Verification items for the finished model (mm, model axes). A direction names the side the tool comes from. Round coordinates to 2 decimals unless told otherwise and drop trailing zeros. Order: outer loops, then holes, each group sorted by start corner. A loop starts at its lowest first (then second) coordinate and runs counter-clockwise, first axis right, second up. Notation, with made-up numbers: (12, -28) -> (62, -28) arc R32 cw to (62, -1) -> close; hole circle Ø4 at (-26, -25). An arc over 180 degrees is marked (long way). Return JSON: item names as keys, results as strings. Group by question number.
Item 1: Sectioned sample at A-A on z = 10. Record the cut outline in (x, y), plus the area to 3 significant figures.
Item 2: Access from +Z, -Z, +X, -X, +Y, -Y to the whole of each face (thin tool, end or side, straight path). Record for faces 5 (the flat face through (-47.5, -90, -31)), 6 (the flat face through (-45, -41, -30)), 7 (the flat face through (47.5, -90, -31)), 8 (the flat face through (0, -95, 1)), 9 (the flat face through (40, -3, -20)).
Item 3: Draft check along X on faces 1 (the flat face through (75, -3, 3)), 2 (the flat face through (-1, -175, -35)), 3 (the flat face through (-1, -172, -35)), 4 (the flat face through (42.5, -79, -27)). Enter one of: pulls with the +X half, pulls with the -X half, needs draft (parallel to the pull), parting line crosses it, or undercut.
Item 4: Depth check by flat-ended pin: pin 1 Ø5.5 at (x, y) = (-46, -58) entering from +Z; pin 2 Ø1.5 at (x, z) = (35, 0) entering from +Y; pin 3 Ø20 at (x, y) = (11.5, -87.5) entering from -Z. Enter the tip coordinate at first touch or a pass-through.
Item 5: Sectioned sample at B-B on y = -98. Record the cut outline in (x, z).
Item 6: Scan lines: probe 1 along X at (y, z) = (-3.8, -32); probe 2 along Z at (x, y) = (-69, -2.2); probe 3 along Y at (x, z) = (45, -11). Record each from-to range of solid material in increasing order. Write a range as from..to.
```python
from build123d import *

# Parameters (mm, degrees)
F0_W     = 5
F0_H     = 3
F0_H_2   = 30
F1_DEPTH = 6
F0_H_3   = 10
F2_DEPTH = 175
F3_DEPTH = 3
F4_START = 172
F0_W_2   = 75
F4_DEPTH = 3
F5_START = 77
F5_DEPTH = 18
F6_D     = 2


# Not quite as in the source:
# - a feature names something its author has since deleted; it is built from what else it names


with BuildPart() as f1:
    # F0 (on Front) → F1 (new body)
    with BuildSketch(Plane.XZ):
        Polygon((75, 48), (-75, 48), (-75, -40), (-47.5, -40), (-47.5, -30), (-47.5, 0), (-47.5, 3), (-42.5, 3), (-42.5, 36), (42.5, 36), (75, 36), align=None)
        Polygon((75, -40), (75, 36), (42.5, 36), (42.5, 3), (47.5, 3), (47.5, 0), (47.5, -30), (47.5, -40), align=None)
        with Locations((45, 1.5)):
            Rectangle(F0_W, F0_H)
        with Locations((45, -15)):
            Rectangle(F0_W, F0_H_2)
        with Locations((-45, 1.5)):
            Rectangle(F0_W, F0_H)
        with Locations((-45, -15)):
            Rectangle(F0_W, F0_H_2)
    extrude(amount=F1_DEPTH)

    # F0 (on Front) → F2 (join)
    with BuildSketch(Plane.XZ):
        with Locations((-45, -35)):
            Rectangle(F0_W, F0_H_3)
        with Locations((45, -35)):
            Rectangle(F0_W, F0_H_3)
    extrude(amount=F2_DEPTH)

    # F0 (on Front) → F3 (join)
    with BuildSketch(Plane.XZ):
        with Locations((-40, -15)):
            Rectangle(F0_W, F0_H_2)
        with Locations((-40, -35)):
            Rectangle(F0_W, F0_H_3)
        with Locations((40, -35)):
            Rectangle(F0_W, F0_H_3)
        with Locations((40, -15)):
            Rectangle(F0_W, F0_H_2)
    extrude(amount=F3_DEPTH)

    # F0 (on Front) → F4 (join)
    with BuildSketch(Plane.XZ.offset(F4_START)):
        with Locations((-40, -35)):
            Rectangle(F0_W, F0_H_3)
        with Locations((40, -35)):
            Rectangle(F0_W, F0_H_3)
        with Locations((0, -35)):
            Rectangle(F0_W_2, F0_H_3)
    extrude(amount=F4_DEPTH)

    # F0 (on Front) → F5 (join)
    with BuildSketch(Plane.XZ.offset(F5_START)):
        with Locations((-45, -15)):
            Rectangle(F0_W, F0_H_2)
        with Locations((45, -15)):
            Rectangle(F0_W, F0_H_2)
        Polygon((42.5, 0), (42.5, 3), (-42.5, 3), (-42.5, 0), (-37.5, 0), (37.5, 0), align=None)
        with Locations((45, 1.5)):
            Rectangle(F0_W, F0_H)
        with Locations((-45, 1.5)):
            Rectangle(F0_W, F0_H)
    extrude(amount=F5_DEPTH)

    # F6 (through all)
    with Locations(Plane(origin=(0, 0, 0), x_dir=(1, 0, 0), z_dir=(0, 1, 0))):
        with Locations((45, -42), (-69, -32), (-69, 32)):
            Hole(F6_D / 2)


solid = f1.part
```
Recorded:
{
 "1": {"outline": "(-75, -6) -> (-42.5, -6) -> (-42.5, 0) -> (-75, 0) -> close; (42.5, -6) -> (75, -6) -> (75, 0) -> (42.5, 0) -> close", "area": "390 mm²"},
 "2": {"face 5": "+Z, -Z, -X, -Y", "face 6": "+Z, +X, -X", "face 7": "+Z, -Z, +X, -Y", "face 8": "+Z, +X, -X, -Y", "face 9": "-Z"},
 "3": {"face 1": "pulls with the +X half", "face 2": "needs draft", "face 3": "undercut", "face 4": "undercut"},
 "4": {"pin 1": "z = -30", "pin 2": "y = -77", "pin 3": "z = 0"},
 "5": {"outline": "(-47.5, -40) -> (-42.5, -40) -> (-42.5, -30) -> (-47.5, -30) -> close; (42.5, -40) -> (47.5, -40) -> (47.5, -30) -> (42.5, -30) -> close"},
 "6": {"probe 1": "-75..-70, -68..-42.5, 42.5..75", "probe 2": "-40..-33, -31..31, 33..48", "probe 3": "-95..-77, -6..0"}
}
